Could you check a few things on this model? Use its own coordinates, in mm. A direction names the side the tool comes from. Give positions to 0.01 mm unless a question says otherwise; leave off trailing zeros. Order: outer loops, then holes, each group sorted by start corner. A loop starts at its lowest first (then second) coordinate and runs counter-clockwise, first axis right, second up. Notation, with made-up numbers: (-32.75, -0.75) - (-24.75, -0.75) arc R28 ccw to (-24.75, 17.25) - close; hole circle Ø8 at (-16.5, 84). An arc over 180 degrees is marked (long way). One line per question, with ' | ' between items. Start each with the question number.
1. Imagine slicing it at A-A (x = -34). Please give me the cut outline in (y, z).
2. Imagine slicing it at B-B (z = 1.1). Please give me the cut outline in (x, y), and give its area (3 significant figures).
3. I need wall thicknesses on probe 1 along Y at (x, z) = (-25, 1.4). Which ranges of the line are inside material? Lowest first, please. Write a range as from..to.
4. Which directions (+Z, -Z, +X, -X, +Y, -Y) give clear straight access to the entire face, cutting with the end or side of a thin tool? Please do faces 5 (the flat face through (-57.938, 36, 1)), 6 (the flat face through (-7.714, 34, 1)).
5. If we mould it in two halves opening along X, with no side actions, what happens to faces 1 (the flat face through (-37, 51.563, 1)), 2 (the flat face through (-15.49, 32, 1)), 3 (the flat face through (-65.714, 34, 1)), 4 (the flat face through (-37, 35.473, 1))? For each: released by +X, released by -X, zero draft, split by the parting line, or undercut.
```python
from build123d import *

# Parameters (mm, degrees)
F0_W     = 58
F0_H     = 35
F0_W_2   = 42.448143
F0_H_2   = 2
F1_DEPTH = 2
F2_R     = 3


with BuildPart() as f1:
    # F0 (on Top) → F1 (new body)
    with BuildSketch(Plane.XY):
        with Locations((-36.713654, 34.063472)):
            Rectangle(F0_W, F0_H)
        with Locations((-36.713654, 31.653472)):
            Rectangle(F0_W_2, F0_H_2, mode=Mode.SUBTRACT)
        with Locations((-36.713654, 36.473472)):
            Rectangle(F0_W_2, F0_H_2, mode=Mode.SUBTRACT)
    extrude(amount=F1_DEPTH)

    # F2
    f2_edges = [f1.edges().sort_by_distance(p)[0] for p in [
        (-7.713654, 51.563472, 1),
        (-65.713654, 16.563472, 1),
        (-65.713654, 51.563472, 1),
        (-7.713654, 16.563472, 1),
    ]]
    fillet(f2_edges, radius=F2_R)


solid = f1.part
```
Results found:
1) outline: (16.56, 0) - (30.65, 0) - (30.65, 2) - (16.56, 2) - close; (32.65, 0) - (35.47, 0) - (35.47, 2) - (32.65, 2) - close; (37.47, 0) - (51.56, 0) - (51.56, 2) - (37.47, 2) - close
2) outline: (-65.71, 19.56) arc R3 ccw to (-62.71, 16.56) - (-10.71, 16.56) arc R3 ccw to (-7.71, 19.56) - (-7.71, 48.56) arc R3 ccw to (-10.71, 51.56) - (-62.71, 51.56) arc R3 ccw to (-65.71, 48.56) - close; hole (-57.94, 30.65) - (-15.49, 30.65) - (-15.49, 32.65) - (-57.94, 32.65) - close; hole (-57.94, 35.47) - (-15.49, 35.47) - (-15.49, 37.47) - (-57.94, 37.47) - close | area: 1,850 mm2
3) probe 1: y = 16.56..30.65, 32.65..35.47, 37.47..51.56
4) face 5: +Z, -Z | face 6: +Z, -Z, +X, +Y, -Y
5) face 1: zero draft | face 2: undercut | face 3: released by -X | face 4: undercut
